The listing builds one solid part. Answer for the finished solid, in the listing's coordinates (mm). Face numbers are marked on the shaded views. Coordinates: 2 decimals unless noted, no trailing zeros.
(1) Straight lines are drawn through the part: line 1 (X direction, y = -45, z = 16); line 2 (Y direction, x = -293, z = 1.5); line 3 (X direction, y = -130, z = -46.5). For each, find the intervals that lie inside material, in ascending order.
(2) For a pull along X with two mould halves and no side action, classify the marked faces 1, 2 and 3 as +X half, -X half, draft (parallel to the pull), parting line (faces both ways), or undercut.
(3) Given P1, Ø12, axis at x = -213.5, y = -99, coming from the +Z side; P2, Ø5, axis at y = -113, z = -36, coming from the +X side; P3, Ø14, axis at y = 3, z = -1, coming from the -X side; P4, Ø1, axis at x = -49, z = 21, coming from the -Y side, each flat-ended and moving along its own axis, determine where each tip first touches the part or whether it passes through.
from build123d import *

# Parameters (mm, degrees)
F3_R = 5.4485927956


with BuildPart() as f1:
    # F0 (on Top) → F1 (revolve)
    with BuildSketch(Plane.XY):
        with BuildLine():
            Line((-76.2, 0), (0, 0))
            Line((0, 0), (0, 50.8))
            Line((0, 50.8), (-19.05, 50.8))
            ThreePointArc((-19.05, 50.8), (-27.6462880029, 46.2224168032), (-33.02, 38.1))
            ThreePointArc((-33.02, 38.1), (-39.9542899622, 32.847360966), (-44.45, 25.4))
            ThreePointArc((-44.45, 25.4), (-51.745724834, 16.4260103223), (-62.1764473617, 11.43))
            Line((-62.1764473617, 11.43), (-62.1764473617, 9.7969081253))
            Line((-62.1764473617, 9.7969081253), (-66.9098570943, 9.7969081253))
            ThreePointArc((-66.9098570943, 9.7969081253), (-71.8643482597, 8.9074053149), (-76.2, 6.35))
            Line((-76.2, 6.35), (-76.2, 0))
        make_face()
    revolve(axis=Axis((-38.1, 0, 0), (-1, 0, 0)))

    # F4: sweep along a path in F2
    with BuildLine(Plane.XY) as f4_path:
        Line((-76.2, 0), (-81.28, 0))
        ThreePointArc((-81.28, 0), (-94.1180458057, 3.4832351865), (-103.4349945345, 12.9775921345))
        ThreePointArc((-103.4349945345, 12.9775921345), (-157.1638386083, 44.45), (-210.892682682, 12.9775921345))
        Line((-210.892682682, 12.9775921345), (-228.6, -18.6028810433))
    # F3 (on face) → F4 (sweep)
    with BuildSketch(Plane(origin=(-76.2, 0, 0), x_dir=(0, -1, 0), z_dir=(-1, 0, 0))):
        Circle(F3_R)
    sweep(path=f4_path.line)

    # F5 (on Top) → F6 (revolve)
    with BuildSketch(Plane.XY):
        Polygon((-189.8287595647, -40.3420948079), (-228.6, -18.6028810433), (-303.134447193, -151.5328482502), (-242.2082122232, -185.6944698804), align=None)
    revolve(axis=Axis((-265.8672235965, -85.0678646468, 0), (-0.4890711758, -0.8722438793, 0)))


solid = f1.part
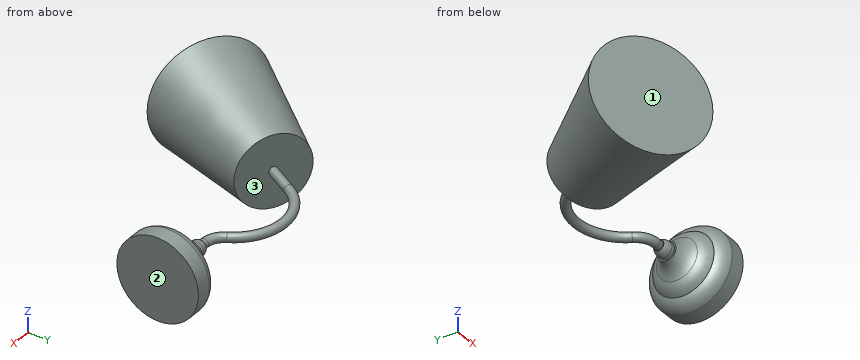
Model answer:
1. line 1: x = -302.95 to -194.55, -25.73 to 0
1. line 2: y = -157.22 to -28.84
1. line 3: x = -341.54 to -244.19
2. face 1: -X half
2. face 2: +X half
2. face 3: undercut
3. P1: stops at z = 29.4
3. P2: stops at x = -227
3. P3: stops at x = -273.09
3. P4: passes through
